Geometry: see drawing. Coordinates: mm, zero at the bounding-box minimum. A direction names the side the tool comes from. Round coordinates to 2 decimals unless told otherwise and drop trailing zeros. Order: outer loops, then holes, each group sorted by start corner. A loop starts at its lowest first (then second) coordinate and runs counter-clockwise, first axis right, second up. Notation, with made-up numbers: (74, 1.25) -> (97, 1.25) arc R13 ccw to (97, 20.25) -> close; hole circle Ø8 at (-6, 8). An arc over 180 degrees is marked (long way). Use a Markdown table: item, result.
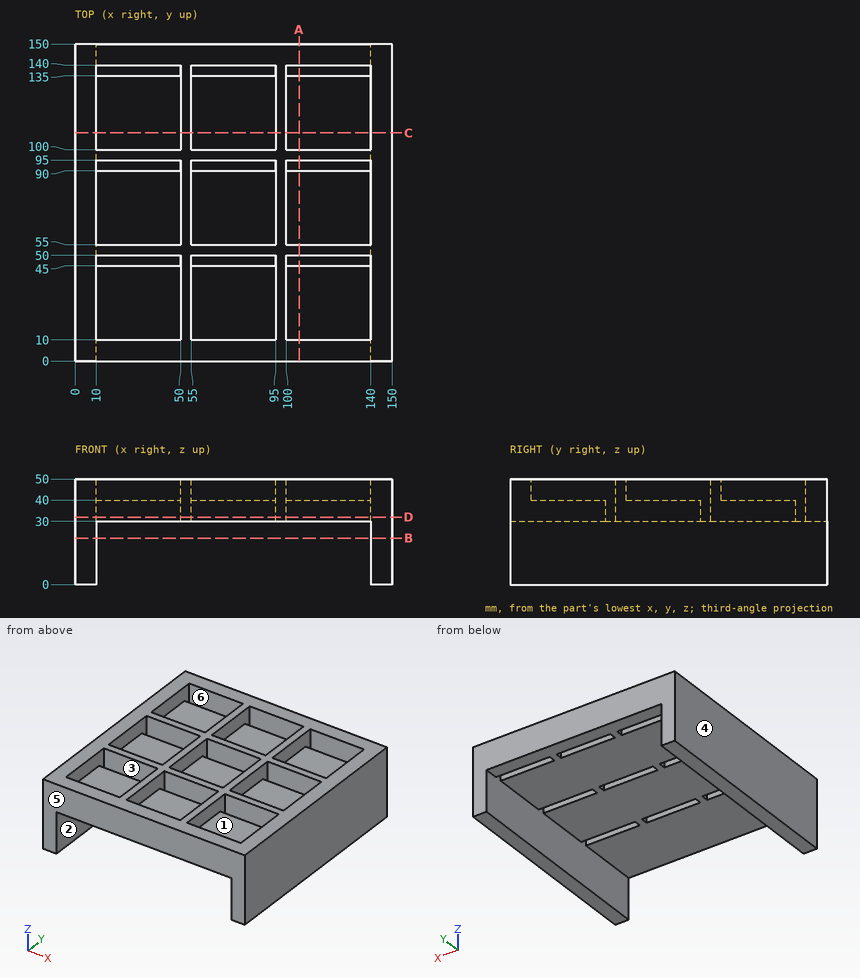
1) Set-up query: the marked faces 1, 2 and 3. Return all of +Z, -Z, +X, -X, +Y, -Y with unobstructed straight access to the full face (end or side cutting, diameter ignored); none if empty.
Answer key:
| item | result |
|---|---|
| face 1 | +Z |
| face 2 | none |
| face 3 | +Z, -Z |
2) Cut plane A-A on x = 106. Return loops of the section in (y, z).
Answer key:
| item | result |
|---|---|
| outline | (0, 30) -> (45, 30) -> (45, 40) -> (10, 40) -> (10, 50) -> (0, 50) -> close; (50, 30) -> (90, 30) -> (90, 40) -> (55, 40) -> (55, 50) -> (50, 50) -> close; (95, 30) -> (135, 30) -> (135, 40) -> (100, 40) -> (100, 50) -> (95, 50) -> close; (140, 30) -> (150, 30) -> (150, 50) -> (140, 50) -> close |
3) Cut plane B-B on z = 22. Return loops of the section in (x, y).
Answer key:
| item | result |
|---|---|
| outline | (0, 0) -> (10, 0) -> (10, 150) -> (0, 150) -> close; (140, 0) -> (150, 0) -> (150, 150) -> (140, 150) -> close |
4) Ray query, probe 1 along Y at (x, z) = (26, 47.5); probe 2 along Y at (x, z) = (73.5, 31.5). Return the intervals inside material, ascending.
Answer key:
| item | result |
|---|---|
| probe 1 | y = 0 to 10, 50 to 55, 95 to 100, 140 to 150 |
| probe 2 | y = 0 to 45, 50 to 90, 95 to 135, 140 to 150 |
5) Contact query for flat-ended pins moving along their axis: P1, Ø17.5, axis at x = 125.5, y = 35.5, coming from the +Z side; P2, Ø1.5, axis at x = 94.5, y = 113, coming from the -Z side. Output: stop coordinate, or through.
Answer key:
| item | result |
|---|---|
| P1 | stops at z = 40 |
| P2 | stops at z = 30 |
6) Draft query along Y for the marked faces 4, 5 and 6. Return one class per face: released by +Y, released by -Y, zero draft, split by the parting line, or undercut.
Answer key:
| item | result |
|---|---|
| face 4 | zero draft |
| face 5 | released by -Y |
| face 6 | undercut |
7) Cut plane D-D on z = 32. State how many separate pieces and enclosed holes the cut face has, and give its area (3 significant figures).
Answer key:
| item | result |
|---|---|
| separate pieces | 1 |
| enclosed holes | 9 |
| area | 20,700 mm^2 |
8) Cut plane C-C on y = 108. Return loops of the section in (x, z), and give its area (3 significant figures).
Answer key:
| item | result |
|---|---|
| outline | (0, 0) -> (10, 0) -> (10, 30) -> (140, 30) -> (140, 0) -> (150, 0) -> (150, 50) -> (140, 50) -> (140, 40) -> (100, 40) -> (100, 50) -> (95, 50) -> (95, 40) -> (55, 40) -> (55, 50) -> (50, 50) -> (50, 40) -> (10, 40) -> (10, 50) -> (0, 50) -> close |
| area | 2,400 mm^2 |
